Verification items for the finished model (mm, model axes). Face numbers are marked on the shaded views. A direction names the side the tool comes from. Round coordinates to 2 decimals unless told otherwise and drop trailing zeros. Loops run counter-clockwise (first coordinate to the right, second up) from the corner with the lowest first, then second, coordinate; pieces in that order, holes last. Notation, with made-up numbers: M 10.5,52 L 68.5,52 A22 cw 68.5,65 Z; hole C 15.5,17 d9. An arc over 180 degrees is marked long. Write item = value, one per line. Start each with the question number.
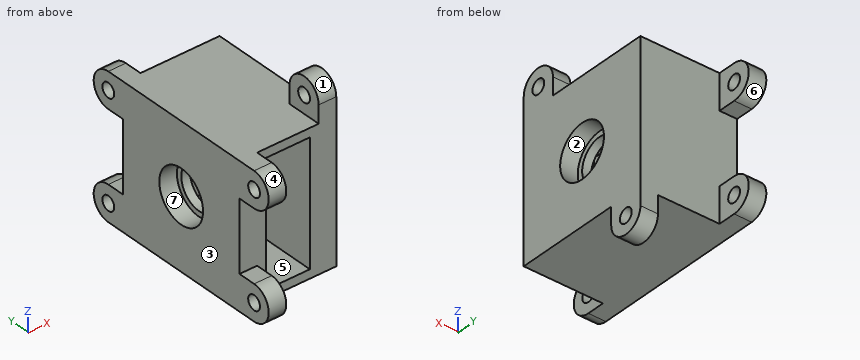
from build123d import *

# Parameters (mm, degrees)
F0_R     = 15
F0_R_2   = 4.05
F1_DEPTH = 10
F2_START = 10
F0_R_3   = 12
F2_DEPTH = 5
F3_START = 15
F3_DEPTH = 25
F4_START = 40
F4_DEPTH = 5
F5_START = 45
F5_DEPTH = 10
F6_START = 45
F6_DEPTH = 10
F7_DEPTH = 10


with BuildPart() as f1:
    # F0 (on Right) → F1 (new body)
    with BuildSketch(Plane.YZ):
        Polygon((35, -40), (40, -40), (40, -20), (40, 20), (40, 25), (40, 35), (40, 40), (-20, 40), (-40, 40), (-40, 35), (35, 35), (35, -35), (-40, -35), (-40, -40), (20, -40), align=None)
        Polygon((-40, -20), (-40, -35), (35, -35), (35, 35), (-40, 35), (-40, 20), align=None)
        Circle(F0_R, mode=Mode.SUBTRACT)
        with BuildLine():
            Line((-50, 20), (-40, 20))
            Line((-40, 20), (-40, 35))
            Line((-40, 35), (-40, 40))
            Line((-40, 40), (-50, 40))
            ThreePointArc((-50, 40), (-60, 30), (-50, 20))
        make_face()
        with Locations((-50, 30)):
            Circle(F0_R_2, mode=Mode.SUBTRACT)
        with BuildLine():
            Line((-50, -40), (-40, -40))
            Line((-40, -40), (-40, -35))
            Line((-40, -35), (-40, -20))
            Line((-40, -20), (-50, -20))
            ThreePointArc((-50, -20), (-60, -30), (-50, -40))
        make_face()
        with Locations((-50, -30)):
            Circle(F0_R_2, mode=Mode.SUBTRACT)
    extrude(amount=F1_DEPTH)

    # F0 (on Right) → F2 (join)
    with BuildSketch(Plane.YZ.offset(F2_START)):
        Polygon((-40, -20), (-40, -35), (35, -35), (35, 35), (-40, 35), (-40, 20), align=None)
        Circle(F0_R, mode=Mode.SUBTRACT)
        Polygon((35, -40), (40, -40), (40, -20), (40, 20), (40, 25), (40, 35), (40, 40), (-20, 40), (-40, 40), (-40, 35), (35, 35), (35, -35), (-40, -35), (-40, -40), (20, -40), align=None)
        Circle(F0_R)
        Circle(F0_R_3, mode=Mode.SUBTRACT)
    extrude(amount=F2_DEPTH)

    # F0 (on Right) → F3 (join)
    with BuildSketch(Plane.YZ.offset(F3_START)):
        Polygon((35, -40), (40, -40), (40, -20), (40, 20), (40, 25), (40, 35), (40, 40), (-20, 40), (-40, 40), (-40, 35), (35, 35), (35, -35), (-40, -35), (-40, -40), (20, -40), align=None)
    extrude(amount=F3_DEPTH)

    # F0 (on Right) → F4 (join)
    with BuildSketch(Plane.YZ.offset(F4_START)):
        Polygon((35, -40), (40, -40), (40, -20), (40, 20), (40, 25), (40, 35), (40, 40), (-20, 40), (-40, 40), (-40, 35), (35, 35), (35, -35), (-40, -35), (-40, -40), (20, -40), align=None)
        Polygon((-40, -20), (-40, -35), (35, -35), (35, 35), (-40, 35), (-40, 20), align=None)
        Circle(F0_R, mode=Mode.SUBTRACT)
        Circle(F0_R)
        Circle(F0_R_3, mode=Mode.SUBTRACT)
    extrude(amount=F4_DEPTH)

    # F0 (on Right) → F5 (join)
    with BuildSketch(Plane.YZ.offset(F5_START)):
        Polygon((35, -40), (40, -40), (40, -20), (40, 20), (40, 25), (40, 35), (40, 40), (-20, 40), (-40, 40), (-40, 35), (35, 35), (35, -35), (-40, -35), (-40, -40), (20, -40), align=None)
        Polygon((-40, -20), (-40, -35), (35, -35), (35, 35), (-40, 35), (-40, 20), align=None)
        Circle(F0_R, mode=Mode.SUBTRACT)
    extrude(amount=F5_DEPTH)

    # F0 (on Right) → F6 (join)
    with BuildSketch(Plane.YZ.offset(F6_START)):
        with BuildLine():
            Line((-40, 40), (-20, 40))
            Line((-20, 40), (-20, 50))
            ThreePointArc((-20, 50), (-30, 60), (-40, 50))
            Line((-40, 50), (-40, 40))
        make_face()
        with Locations((-30, 50)):
            Circle(F0_R_2, mode=Mode.SUBTRACT)
        with BuildLine():
            Line((40, -50), (40, -40))
            Line((40, -40), (35, -40))
            Line((35, -40), (20, -40))
            Line((20, -40), (20, -50))
            ThreePointArc((20, -50), (30, -60), (40, -50))
        make_face()
        with Locations((30, -50)):
            Circle(F0_R_2, mode=Mode.SUBTRACT)
    extrude(amount=F6_DEPTH)

    # F0 (on Right) → F7 (join)
    with BuildSketch(Plane.YZ):
        with BuildLine():
            Line((40, 25), (40, 20))
            Line((40, 20), (50, 20))
            ThreePointArc((50, 20), (60, 30), (50, 40))
            Line((50, 40), (40, 40))
            Line((40, 40), (40, 35))
            Line((40, 35), (40, 25))
        make_face()
        with Locations((50, 30)):
            Circle(F0_R_2, mode=Mode.SUBTRACT)
        with BuildLine():
            Line((40, -20), (40, -40))
            Line((40, -40), (50, -40))
            ThreePointArc((50, -40), (60, -30), (50, -20))
            Line((50, -20), (40, -20))
        make_face()
        with Locations((50, -30)):
            Circle(F0_R_2, mode=Mode.SUBTRACT)
    extrude(amount=F7_DEPTH)


solid = f1.part
1. Thickness scan on line 1 (Z direction, x = 3, y = -50); line 2 (Z direction, x = 47.5, y = 30); line 3 (Z direction, x = 22.5, y = -18.5). Record the ranges inside material, lowest first.
2. Gauge pin test, flat ends, axial feed: P1, Ø4, axis at x = 45, y = 0.5, coming from the +Z side; P2, Ø10, axis at x = 31.5, z = 29.5, coming from the -Y side; P3, Ø3, axis at x = 8, z = 34.5, coming from the +Y side; P4, Ø22, axis at y = -49.5, z = 32.5, coming from the +X side. Record the tip position at first contact, or that the pin passes through.
3. Mould release check, pull along Y, two halves, no side actions. Record for the marked faces 1, 2, 3 and 4: pulls with the +Y half, pulls with the -Y half, needs draft (parallel to the pull), parting line crosses it, or undercut.
4. Section check D-D, the plane y = 0. Enter the section's corners in (x, z).
5. Tool access check on the marked faces 5, 6 and 7. Record the directions out of +Z, -Z, +X, -X, +Y, -Y that give a thin tool (end or side, any length) a straight path to the whole face; none if there is none.
6. Section check B-B, the plane x = 48.5. Enter the section's corners in (y, z), and give its area (3 significant figures).
7. Section check C-C, the plane z = 30. Enter the section's corners in (x, y), and give its area (3 significant figures).
8. Section check A-A, the plane y = 30. Enter the section's corners in (x, z), and give its area (3 significant figures).
Computed values:
q1.line_1 = -40 to -34.05, -25.95 to -20, 20 to 25.95, 34.05 to 40
q1.line_2 = -60 to -54.05, -45.95 to 40
q1.line_3 = -40 to -35, 35 to 40
q2.P1 = 40
q2.P2 = 35
q2.P3 = 59.54
q2.P4 = 55
q3.face_1 = parting line crosses it
q3.face_2 = undercut
q3.face_3 = needs draft
q3.face_4 = pulls with the -Y half
q4.outline = M 0,-40 L 55,-40 L 55,-15 L 45,-15 L 45,-12 L 40,-12 L 40,-35 L 15,-35 L 15,-12 L 10,-12 L 10,-15 L 0,-15 Z; M 0,15 L 10,15 L 10,12 L 15,12 L 15,35 L 40,35 L 40,12 L 45,12 L 45,15 L 55,15 L 55,40 L 0,40 Z
q5.face_5 = -Y
q5.face_6 = +X, -X, +Y
q5.face_7 = -X
q6.outline = M -40,-40 L 20,-40 L 20,-50 A10 ccw 40,-50 L 40,40 L -20,40 L -20,50 A10 ccw -40,50 Z; hole C -30,50 d8.1; hole C 0,0 d30; hole C 30,-50 d8.1
q6.area = 6,300 mm2
q7.outline = M 0,-60 L 10,-60 L 10,-54.05 L 0,-54.05 Z; M 0,-45.95 L 10,-45.95 L 10,-40 L 15,-40 L 15,35 L 40,35 L 40,-40 L 55,-40 L 55,40 L 10,40 L 10,45.95 L 0,45.95 Z; M 0,54.05 L 10,54.05 L 10,60 L 0,60 Z
q7.area = 2,760 mm2
q8.outline = M 0,-40 L 45,-40 L 45,-45.95 L 55,-45.95 L 55,40 L 0,40 Z; M 45,-60 L 55,-60 L 55,-54.05 L 45,-54.05 Z; hole M 15,-35 L 40,-35 L 40,35 L 15,35 Z
q8.area = 2,770 mm2
